Check sheet for the modelled part. Datum: model origin and axes. Units: mm. A direction names the side the tool comes from. Coordinates: 2 decimals unless noted, no trailing zeros. Order: outer loops, then holes, each group sorted by start corner. A loop starts at its lowest first (then second) coordinate and runs counter-clockwise, first axis right, second up.
from build123d import *

# Parameters (mm, degrees)
SKETCH1_W           = 40
SKETCH1_H           = 40
SKETCH1_W_2         = 32
SKETCH1_H_2         = 32
BOSS_EXTRUDE1_DEPTH = 900
CUT_EXTRUDE1_DEPTH  = 20
SKETCH3_R           = 6.1
CUT_EXTRUDE2_DEPTH  = 20
SKETCH4_R           = 6.1
CUT_EXTRUDE3_DEPTH  = 20
SKETCH5_R           = 6.1
CUT_EXTRUDE4_DEPTH  = 60
SKETCH6_R           = 6.1
CUT_EXTRUDE5_DEPTH  = 60


with BuildPart() as part:
    # Sketch1 → Boss-Extrude1 (new body)
    with BuildSketch(Plane.XY):
        Rectangle(SKETCH1_W, SKETCH1_H)
        Rectangle(SKETCH1_W_2, SKETCH1_H_2, mode=Mode.SUBTRACT)
    extrude(amount=BOSS_EXTRUDE1_DEPTH)

    # Sketch2 → Cut-Extrude1 (cut)
    with BuildSketch(Plane(origin=(0, 0, 0), x_dir=(-1, 0, 0), z_dir=(0, 0, -1))):
        Polygon((-16, -16), (-16, -20), (20, -20), (20, 16), (16, 16), (16, -16), align=None)
    extrude(amount=-CUT_EXTRUDE1_DEPTH, mode=Mode.SUBTRACT)

    # Sketch3 → Cut-Extrude2 (cut)
    with BuildSketch(Plane.ZY.offset(-16)):
        with Locations(Location((10, -4, 0), (0, 0, 270))):
            Circle(SKETCH3_R)
    extrude(amount=-CUT_EXTRUDE2_DEPTH, mode=Mode.SUBTRACT)

    # Sketch4 → Cut-Extrude3 (cut)
    with BuildSketch(Plane.XZ.offset(-16)):
        with Locations((-4, 10)):
            Circle(SKETCH4_R)
    extrude(amount=-CUT_EXTRUDE3_DEPTH, mode=Mode.SUBTRACT)

    # Sketch5 → Cut-Extrude4 (cut)
    with BuildSketch(Plane.XZ.offset(20)):
        with Locations(Location((0, 890, 0), (0, 0, 270))):
            Circle(SKETCH5_R)
    extrude(amount=-CUT_EXTRUDE4_DEPTH, mode=Mode.SUBTRACT)

    # Sketch6 → Cut-Extrude5 (cut)
    with BuildSketch(Plane.ZY.offset(20)):
        with Locations((890, 0)):
            Circle(SKETCH6_R)
    extrude(amount=-CUT_EXTRUDE5_DEPTH, mode=Mode.SUBTRACT)


solid = part.part
(1) Release check for a two-part mould opening along X. For faces 1 (the flat face through (-20, 0, 444)), 2 (the flat face through (-2, 16, 444)), 3 (the flat face through (0, -20, 444)), 4 (the flat face through (20, 0, 444)) record: +X half, -X half, draft (parallel to the pull), parting line (faces both ways), or undercut.
Filled in:
face 1: -X half
face 2: undercut
face 3: draft
face 4: +X half
(2) Cross-section at A-A (z = 414). Enter the section's corners in (x, y), and give its area (3 significant figures).
Filled in:
outline: (-20, -20) - (20, -20) - (20, 20) - (-20, 20) - close; hole (-16, -16) - (16, -16) - (16, 16) - (-16, 16) - close
area: 576 mm2
(3) Tool access check on faces 5 (the flat face through (7.3, 16.4, 0)), 6 (the flat face through (-10, -17, 20)), 7 (the flat face through (0, -16, 454)). Record the directions out of +Z, -Z, +X, -X, +Y, -Y that give a thin tool (end or side, any length) a straight path to the whole face; none if there is none.
Filled in:
face 5: -Z, +X, -X, +Y, -Y
face 6: -Z, -X, -Y
face 7: +Z, -Z
(4) Thickness scan on probe 1 along Y at (x, z) = (-17.5, 890); probe 2 along X at (y, z) = (-12, 278). Record the ranges inside material, lowest first.
Filled in:
probe 1: y = -20 to -6.1, 6.1 to 20
probe 2: x = -20 to -16, 16 to 20
(5) Go/stop test with flat-tipped pins: P1, Ø4, axis at x = 15, y = 10, coming from the -Z side; P2, Ø5, axis at x = 12, y = -7, coming from the -Z side; P3, Ø14, axis at y = -4, z = 10, coming from the -X side. Record where each tip stops, or that it passes through.
Filled in:
P1: stops at z = 0
P2: passes through
P3: stops at x = 16
